```python
from build123d import *

# Parameters (mm, degrees)
SKETCH_1_W          = 162
SKETCH_1_H          = 111
EXTRUDE_1_DEPTH     = 5
CUT_EXTRUDE_1_REACH = 198.443
SKETCH_2_W          = 20
SKETCH_2_H          = 82
SKETCH_3_R          = 1.5
SKETCH_3_R_2        = 1
SKETCH_3_R_3        = 2.5
SKETCH_3_W          = 7
SKETCH_3_H          = 60
CUT_EXTRUDE_2_DEPTH = 5
FILLET_1_R          = 3
SKETCH1_W           = 5
SKETCH1_H           = 15
BOSS_EXTRUDE1_DEPTH = 6
SKETCH2_W           = 12
SKETCH2_H           = 24
BOSS_EXTRUDE2_DEPTH = 5
SKETCH3_W           = 5
SKETCH3_H           = 2
CUT_EXTRUDE2_DEPTH  = 197.443376065
FILLET1_R           = 3


with BuildPart() as part:
    # 草图1 → 凸台-拉伸1 (new body)
    with BuildSketch(Plane.XY):
        with Locations((81, -55.5)):
            Rectangle(SKETCH_1_W, SKETCH_1_H)
    extrude(amount=EXTRUDE_1_DEPTH)

    # 草图2 → 切除-拉伸1 (cut, up to next)
    with BuildSketch(Plane(origin=(0, 0, 0), x_dir=(-1, 0, 0), z_dir=(0, 0, -1)), mode=Mode.PRIVATE) as cut_extrude_1_sk1:
        with Locations((-120, -55.5)):
            Rectangle(SKETCH_2_W, SKETCH_2_H)
    cut_extrude_1_tool1 = extrude(cut_extrude_1_sk1.sketch, amount=-CUT_EXTRUDE_1_REACH, mode=Mode.PRIVATE) & part.part
    add(cut_extrude_1_tool1.solids().sort_by_distance((120, -55.5, 0))[0], mode=Mode.SUBTRACT)

    # 草图3 → 切除-拉伸2 (cut)
    with BuildSketch(Plane.XY.offset(5)):
        with Locations((149, -60.5)):
            Circle(SKETCH_3_R)
        with Locations((139, -60.5)):
            Circle(SKETCH_3_R)
        with Locations((149, -91.5)):
            Circle(SKETCH_3_R)
        with Locations((139, -91.5)):
            Circle(SKETCH_3_R)
        with Locations((149, -50.5)):
            Circle(SKETCH_3_R)
        with Locations((139, -50.5)):
            Circle(SKETCH_3_R)
        with Locations((22.5, -103)):
            Circle(SKETCH_3_R_2)
        with Locations((22.5, -8)):
            Circle(SKETCH_3_R_2)
        with Locations((21, -60.5)):
            Circle(SKETCH_3_R)
        with Locations((21, -91.5)):
            Circle(SKETCH_3_R)
        with Locations((21, -50.5)):
            Circle(SKETCH_3_R)
        with Locations((21, -19.5)):
            Circle(SKETCH_3_R)
        with Locations((10, -8)):
            Circle(SKETCH_3_R_3)
        with Locations((152, -8)):
            Circle(SKETCH_3_R_3)
        with Locations((152, -103)):
            Circle(SKETCH_3_R_3)
        with Locations((10, -103)):
            Circle(SKETCH_3_R_3)
        with Locations((37.5, -103)):
            Circle(SKETCH_3_R_2)
        with Locations((52.5, -103)):
            Circle(SKETCH_3_R_2)
        with Locations((67.5, -103)):
            Circle(SKETCH_3_R_2)
        with Locations((82.5, -103)):
            Circle(SKETCH_3_R_2)
        with Locations((97.5, -103)):
            Circle(SKETCH_3_R_2)
        with Locations((37.5, -8)):
            Circle(SKETCH_3_R_2)
        with Locations((52.5, -8)):
            Circle(SKETCH_3_R_2)
        with Locations((67.5, -8)):
            Circle(SKETCH_3_R_2)
        with Locations((82.5, -8)):
            Circle(SKETCH_3_R_2)
        with Locations((97.5, -8)):
            Circle(SKETCH_3_R_2)
        with Locations((112.5, -8)):
            Circle(SKETCH_3_R_2)
        with Locations((139, -19.5)):
            Circle(SKETCH_3_R)
        with Locations((149, -19.5)):
            Circle(SKETCH_3_R)
        with Locations((112.5, -103)):
            Circle(SKETCH_3_R_2)
        with Locations((52.5, -55.5)):
            Circle(SKETCH_3_R)
        with Locations((97.5, -55.5)):
            Circle(SKETCH_3_R)
        with Locations((8.5, -55.5)):
            Rectangle(SKETCH_3_W, SKETCH_3_H)
    extrude(amount=-CUT_EXTRUDE_2_DEPTH, mode=Mode.SUBTRACT)

    # 圆角1
    fillet_1_edges = [part.edges().sort_by_distance(p)[0] for p in [
        (5, -25.5, 2.5),
        (12, -25.5, 2.5),
        (12, -85.5, 2.5),
        (5, -85.5, 2.5),
        (110, -96.5, 2.5),
        (130, -96.5, 2.5),
        (130, -14.5, 2.5),
        (110, -14.5, 2.5),
        (0, 0, 2.5),
        (162, 0, 2.5),
        (162, -111, 2.5),
        (0, -111, 2.5),
    ]]
    fillet(fillet_1_edges, radius=FILLET_1_R)

    # Sketch1 → Boss-Extrude1 (add)
    with BuildSketch(Plane.ZY):
        with Locations((2.5, -90.5)):
            Rectangle(SKETCH1_W, SKETCH1_H)
        with Locations((2.5, -20.5)):
            Rectangle(SKETCH1_W, SKETCH1_H)
    extrude(amount=BOSS_EXTRUDE1_DEPTH)

    # Sketch2 → Boss-Extrude2 (add)
    with BuildSketch(Plane.XY):
        with Locations((6, -55.5)):
            Rectangle(SKETCH2_W, SKETCH2_H)
    extrude(amount=BOSS_EXTRUDE2_DEPTH)

    # Sketch3 → Cut-Extrude2 (cut, through all)
    with BuildSketch(Plane.XY):
        with Locations((2.5, -35.5)):
            Rectangle(SKETCH3_W, SKETCH3_H)
        with Locations((2.5, -75.5)):
            Rectangle(SKETCH3_W, SKETCH3_H)
    extrude(amount=CUT_EXTRUDE2_DEPTH, mode=Mode.SUBTRACT)

    # Fillet1
    fillet1_edges = [part.edges().sort_by_distance(p)[0] for p in [
        (-6, -13, 2.5),
        (-6, -28, 2.5),
        (-6, -98, 2.5),
        (-6, -83, 2.5),
        (5, -67.5, 2.5),
        (5, -43.5, 2.5),
        (12, -43.5, 2.5),
        (12, -67.5, 2.5),
    ]]
    fillet(fillet1_edges, radius=FILLET1_R)


solid = part.part
```
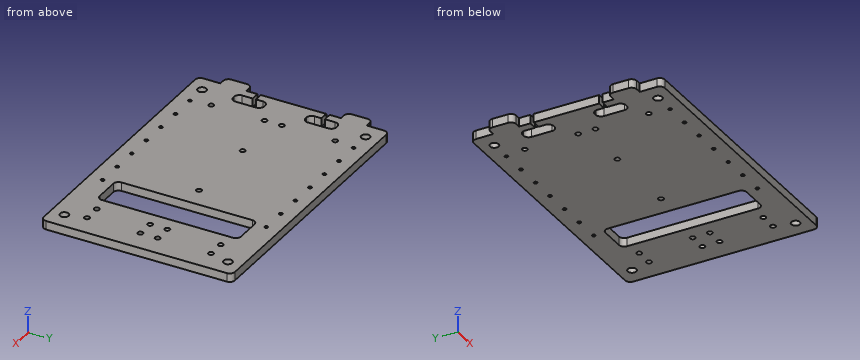
For this review, take the finished solid that the model builds, in its own axes (mm). Coordinates: 2 decimals unless noted, no trailing zeros. Write each loop counter-clockwise with the first axis right and the second up, starting at its lowest first coordinate (ties: lowest second). Pieces come first, ordered by that corner, then holes.
(1) For pin 1 Ø1.5 at (y, z) = (-30, 2.5) entering from -X; pin 2 Ø1.6 at (x, y) = (112.5, -103) entering from -Z; pin 3 Ø2.5 at (x, z) = (-1.5, 3.5) entering from +Y, all flat-tipped, find the tip position at first contact; note any pin that passes through.
(2) Add section B-B on z = 1. Count the separate pieces of the cut face and the enclosed holes in it, then the cut area to 3 significant figures.
(3) Wall thickness on probe 1 along Y at (x, z) = (37.5, 2.3); probe 2 along Y at (x, z) = (149, 1.85); probe 3 along Y at (x, z) = (97.5, 1.75): over which ranges is each line inside the solid? List them lowest first.
(4) Add section A-A on y = -80. Give the boundary of the cut face in (x, z), then the cut area to 3 significant figures.
Answer sheet:
1. pin 1: stops at x = 0
1. pin 2: passes through
1. pin 3: stops at y = -13
2. separate pieces: 1
2. enclosed holes: 33
2. area: 16,000 mm2
3. probe 1: y = -111 to -104, -102 to -9, -7 to 0
3. probe 2: y = -111 to -93, -90 to -62, -59 to -52, -49 to -21, -18 to 0
3. probe 3: y = -111 to -104, -102 to -57, -54 to -9, -7 to 0
4. outline: (0, 0) - (5, 0) - (5, 5) - (0, 5) - close; (12, 0) - (110, 0) - (110, 5) - (12, 5) - close; (130, 0) - (162, 0) - (162, 5) - (130, 5) - close
4. area: 675 mm2
